```python
from build123d import *

# Parameters (mm, degrees)
F0_W     = 200
F0_H     = 100
F1_DEPTH = 15
F2_W     = 10
F2_H     = 10
F3_DEPTH = 50
F4_W     = 50
F4_H     = 6
F5_DEPTH = 10


# Not quite as in the source:
# - a feature names something its author has since deleted; it is built from what else it names


with BuildPart() as f1:
    # F0 (on Front) → F1 (new body)
    with BuildSketch(Plane.XZ):
        with Locations((46.1999992281, 49.9613083565)):
            Rectangle(F0_W, F0_H)
    extrude(amount=F1_DEPTH)

    # F2 (on face) → F3 (join)
    with BuildSketch(Plane.XZ.offset(15)):
        with Locations((-43.8000007719, 89.9613083565)):
            Rectangle(F2_W, F2_H)
        with Locations((-43.8000007719, 9.9613083565)):
            Rectangle(F2_W, F2_H)
        with Locations((136.1999992281, 89.9613083565)):
            Rectangle(F2_W, F2_H)
        with Locations((136.1999992281, 9.9613083565)):
            Rectangle(F2_W, F2_H)
    extrude(amount=F3_DEPTH)

    # F4 (on face) → F5 (cut, symmetric)
    with BuildSketch(Plane.XY.offset(94.9613083565)):
        with Locations((25, -6.6546534393)):
            Rectangle(F4_W, F4_H)
    extrude(amount=F5_DEPTH, both=True, mode=Mode.SUBTRACT)


solid = f1.part
```
Part model, mm, in its own coordinate system. A direction names the side the tool comes from. Round coordinates to 2 decimals unless told otherwise and drop trailing zeros. Loops run counter-clockwise (first coordinate to the right, second up) from the corner with the lowest first, then second, coordinate; pieces in that order, holes last. Notation, with made-up numbers: (29.25, 26.5) -> (65.25, 26.5) arc R11 ccw to (65.25, 33.5) -> close; hole circle Ø3 at (-6, 36.5). An arc over 180 degrees is marked (long way). Use one line per item in the form item = value. Start each with the question number.
Item 1: Band-saw the part on A-A (y = -18). List the corners of the cut face in (x, z).
Item 2: Band-saw the part on D-D (z = 36.5). List the corners of the cut face in (x, y).
Item 3: Drop flat-ended pins along their axis: pin 1 Ø11 at (x, y) = (-44.5, -48.5) entering from -Z; pin 2 Ø3 at (y, z) = (-52, 8) entering from +X; pin 3 Ø3 at (y, z) = (-45, 12.5) entering from -X. Give the stop position or say it passes through.
Item 4: Two-plate mould, pull along Z, no slides. Class faces 6 (the flat face through (136, -40, 94.961)), 7 (the flat face through (136, -40, 84.961)), 8 (the flat face through (0, -7, 93)): released by +Z, released by -Z, zero draft, split by the parting line, or undercut.
Item 5: Tool access for faces 1 (the flat face through (-44, -40, 14.961)), 2 (the flat face through (25, -9.655, 93)), 3 (the flat face through (-44, -40, 4.961)), 4 (the flat face through (-38.8, -40, 90)), 5 (the flat face through (-48.8, -40, 90)): list every direction of +Z, -Z, +X, -X, +Y, -Y with a clear straight run to the whole face (end or side of a thin tool).
Item 6: Drill centre lines: line 1 along X through (y, z) = (-25.5, 13); line 2 along X through (y, z) = (-9, 85.5); line 3 along Y through (x, z) = (-16.5, 28.5). Where is each one in solid material? Low to high.
Item 7: Band-saw the part on B-B (z = 89.5). List the corners of the cut face in (x, y), plus the area to 3 significant figures.
Item 8: Band-saw the part on C-C (x = 28). List the corners of the cut face in (y, z).
Data:
q1.outline = (-48.8, 4.96) -> (-38.8, 4.96) -> (-38.8, 14.96) -> (-48.8, 14.96) -> close; (-48.8, 84.96) -> (-38.8, 84.96) -> (-38.8, 94.96) -> (-48.8, 94.96) -> close; (131.2, 4.96) -> (141.2, 4.96) -> (141.2, 14.96) -> (131.2, 14.96) -> close; (131.2, 84.96) -> (141.2, 84.96) -> (141.2, 94.96) -> (131.2, 94.96) -> close
q2.outline = (-53.8, -15) -> (146.2, -15) -> (146.2, 0) -> (-53.8, 0) -> close
q3.pin_1 = 4.96
q3.pin_2 = 141.2
q3.pin_3 = -48.8
q4.face_6 = released by +Z
q4.face_7 = undercut
q4.face_8 = zero draft
q5.face_1 = +X, -X, -Y
q5.face_2 = +Z
q5.face_3 = -Z, +X, -X, -Y
q5.face_4 = +Z, -Z, -Y
q5.face_5 = +Z, -Z, -X, -Y
q6.line_1 = -48.8 to -38.8, 131.2 to 141.2
q6.line_2 = -53.8 to 0, 50 to 146.2
q6.line_3 = -15 to 0
q7.outline = (-53.8, -15) -> (-48.8, -15) -> (-48.8, -65) -> (-38.8, -65) -> (-38.8, -15) -> (131.2, -15) -> (131.2, -65) -> (141.2, -65) -> (141.2, -15) -> (146.2, -15) -> (146.2, 0) -> (-53.8, 0) -> close; hole (0, -9.65) -> (50, -9.65) -> (50, -3.65) -> (0, -3.65) -> close
q7.area = 3,700 mm^2
q8.outline = (-15, -0.04) -> (0, -0.04) -> (0, 99.96) -> (-3.65, 99.96) -> (-3.65, 84.96) -> (-9.65, 84.96) -> (-9.65, 99.96) -> (-15, 99.96) -> close
